Geometry check sheet. Reference: the model listing, model coordinates, mm. A direction names the side the tool comes from. Coordinates: 2 decimals unless noted, no trailing zeros. Write each loop counter-clockwise with the first axis right and the second up, starting at its lowest first coordinate (ties: lowest second). Pieces come first, ordered by that corner, then holes. Notation, with made-up numbers: (40.5, 50.25) -> (62.5, 50.25) arc R29 cw to (62.5, 78.25) -> close; hole circle Ø6 at (-25, 78). An arc over 180 degrees is marked (long way). Use a Markdown table: item, result.
```python
from build123d import *

# Parameters (mm, degrees)
F0_R     = 5.55625
F0_R_2   = 2.8575
F1_DEPTH = 3.175
F2_W     = 1.5875
F2_H     = 0.80645


with BuildPart() as f1:
    # F0 (on Right) → F1 (new body)
    with BuildSketch(Plane.YZ):
        Circle(F0_R)
        Circle(F0_R_2, mode=Mode.SUBTRACT)
    extrude(amount=F1_DEPTH)

    # F2 (on Front) → F3 (revolve, cut)
    with BuildSketch(Plane.XZ):
        with Locations((1.5875, 5.153025)):
            Rectangle(F2_W, F2_H)
    revolve(axis=Axis((-3.449974, 0, 0), (-1, 0, 0)), mode=Mode.SUBTRACT)


solid = f1.part
```
Item 1: Section check D-D on z = 4. Record the boundary of the cut face in (x, y) (3 decimals).
Answer block:
| item | result |
|---|---|
| outline | (0, -3.856) -> (0.794, -3.856) -> (0.794, -2.561) -> (2.381, -2.561) -> (2.381, -3.856) -> (3.175, -3.856) -> (3.175, 3.856) -> (2.381, 3.856) -> (2.381, 2.561) -> (0.794, 2.561) -> (0.794, 3.856) -> (0, 3.856) -> close |
Item 2: Thickness scan on L1, parallel to X at y = -4.5, z = 3 (3 decimals); L2, parallel to Y at x = 1.6, z = -1.5; L3, parallel to Z at x = 0.95, y = -0.75. Record the ranges inside material, lowest first. Write a range as [from, to].
Answer block:
| item | result |
|---|---|
| L1 | x = [0, 0.794], [2.381, 3.175] |
| L2 | y = [-4.51, -2.43], [2.43, 4.51] |
| L3 | z = [-4.69, -2.76], [2.76, 4.69] |
Item 3: Depth check by flat-ended pin: P1, Ø5, axis at y = 0, z = 0, coming from the +X side. Enter the tip coordinate at first touch or a pass-through.
Answer block:
| item | result |
|---|---|
| P1 | passes through |
Item 4: Section check A-A on z = 0. Record the boundary of the cut face in (x, y) (1 decimal), then the cut area to 3 significant figures.
Answer block:
| item | result |
|---|---|
| outline | (0, -5.6) -> (0.8, -5.6) -> (0.8, -4.7) -> (2.4, -4.7) -> (2.4, -5.6) -> (3.2, -5.6) -> (3.2, -2.9) -> (0, -2.9) -> close; (0, 2.9) -> (3.2, 2.9) -> (3.2, 5.6) -> (2.4, 5.6) -> (2.4, 4.7) -> (0.8, 4.7) -> (0.8, 5.6) -> (0, 5.6) -> close |
| area | 14.6 mm^2 |
Item 5: Mould release check, pull along Y, two halves, no side actions. Record for faces 1 (the cylindrical face through (0.39, 5.3, 1.67)), 2 (the flat face through (3.175, -3, 1)), 3 (the cylindrical face through (1.565, 2.726, 0.858)): +Y half, -Y half, draft (parallel to the pull), parting line (faces both ways), or undercut.
Answer block:
| item | result |
|---|---|
| face 1 | parting line |
| face 2 | draft |
| face 3 | undercut |
Item 6: Tool access check on faces 4 (the cylindrical face through (2.77, 5.3, 1.67)), 5 (the flat face through (0.794, 2, -5)). Record the directions out of +Z, -Z, +X, -X, +Y, -Y that give a thin tool (end or side, any length) a straight path to the whole face; none if there is none.
Answer block:
| item | result |
|---|---|
| face 4 | +X, -X |
| face 5 | none |
Item 7: Section check C-C on x = 0.3. Record the boundary of the cut face in (y, z) (1 decimal).
Answer block:
| item | result |
|---|---|
| outline | circle Ø11.1 at (0, 0); hole circle Ø5.7 at (0, 0) |
